Part model, mm, in its own coordinate system. Face numbers are marked on the shaded views. A direction names the side the tool comes from. Give positions to 0.01 mm unless a question says otherwise; leave off trailing zeros. Order: outer loops, then holes, each group sorted by start corner. A loop starts at its lowest first (then second) coordinate and runs counter-clockwise, first axis right, second up. Notation, with made-up numbers: (20.25, -6) - (27.25, -6) arc R20 cw to (27.25, 15) - close; hole circle Ø2 at (-33, 80). An arc over 180 degrees is marked (long way). Use a Markdown table: item, result. Add a question column.
from build123d import *

# Parameters (mm, degrees)
SKETCH1_R           = 127
BOSS_EXTRUDE1_DEPTH = 63.5
BOSS_EXTRUDE2_DEPTH = 381
CUT_EXTRUDE1_DEPTH  = 203.2
CUT_EXTRUDE2_DEPTH  = 203.2
FILLET1_R           = 25.4
FILLET2_R           = 25.4
FILLET3_R           = 25.4
SKETCH5_R           = 127
BOSS_EXTRUDE3_DEPTH = 304.8
SKETCH6_R           = 63.5
BOSS_EXTRUDE4_DEPTH = 127


with BuildPart() as part:
    # Sketch1 → Boss-Extrude1 (new body, symmetric)
    with BuildSketch(Plane(origin=(0, 0, 0), x_dir=(0, 0, -1), z_dir=(1, 0, 0))):
        Circle(SKETCH1_R)
    extrude(amount=BOSS_EXTRUDE1_DEPTH, both=True)

    # Sketch2 → Boss-Extrude2 (add, symmetric)
    with BuildSketch(Plane.XY):
        Polygon((88.9, -120.65), (88.9, 120.65), (317.5, 158.75), (311.236398584, 196.331608498), (50.8, 152.925542067), (50.8, -152.925542067), (311.236398584, -196.331608498), (317.5, -158.75), align=None)
    extrude(amount=BOSS_EXTRUDE2_DEPTH, both=True)

    # Sketch3 → Cut-Extrude1 (cut)
    with BuildSketch(Plane(origin=(334.662162162, 55.777027027, 0), x_dir=(0, 0, -1), z_dir=(0.986393924, 0.164398987, 0))):
        Polygon((0, 104.393356939), (-127, 104.393356939), (-127, 142.493356939), (127, 142.493356939), (127, 104.393356939), align=None)
    extrude(amount=-CUT_EXTRUDE1_DEPTH, mode=Mode.SUBTRACT)

    # Sketch4 → Cut-Extrude2 (cut)
    with BuildSketch(Plane(origin=(334.662162162, -55.777027027, 0), x_dir=(0, 0, -1), z_dir=(0.986393924, -0.164398987, 0))):
        Polygon((0, -142.493356939), (-127, -142.493356939), (-127, -104.393356939), (127, -104.393356939), (127, -142.493356939), align=None)
    extrude(amount=-CUT_EXTRUDE2_DEPTH, mode=Mode.SUBTRACT)

    # Fillet1
    fillet1_edges = [part.edges().sort_by_distance(p)[0] for p in [
        (88.9, -120.65, 0),
        (88.9, 120.65, 0),
    ]]
    fillet(fillet1_edges, radius=FILLET1_R)

    # Fillet2
    fillet2_edges = [part.edges().sort_by_distance(p)[0] for p in [
        (50.8, 152.925542067, 0),
        (50.8, -152.925542067, 0),
    ]]
    fillet(fillet2_edges, radius=FILLET2_R)

    # Fillet3
    fillet3_edges = [part.edges().sort_by_distance(p)[0] for p in [
        (314.368199292, -177.540804249, 381),
        (113.932953969, 144.134930029, 127),
        (113.932953969, 144.134930029, -127),
        (314.368199292, 177.540804249, -127),
        (314.368199292, 177.540804249, 127),
        (113.932953969, -144.134930029, 127),
        (113.932953969, -144.134930029, -127),
        (314.368199292, -177.540804249, -127),
        (314.368199292, -177.540804249, 127),
        (314.368199292, 177.540804249, -381),
        (314.368199292, -177.540804249, -381),
        (314.368199292, 177.540804249, 381),
    ]]
    fillet(fillet3_edges, radius=FILLET3_R)

    # Sketch5 → Boss-Extrude3 (add)
    with BuildSketch(Plane.ZY.offset(63.5)):
        Circle(SKETCH5_R)
    extrude(amount=BOSS_EXTRUDE3_DEPTH)

    # Sketch6 → Boss-Extrude4 (add)
    with BuildSketch(Plane.ZY.offset(368.3)):
        Circle(SKETCH6_R)
    extrude(amount=BOSS_EXTRUDE4_DEPTH)


solid = part.part
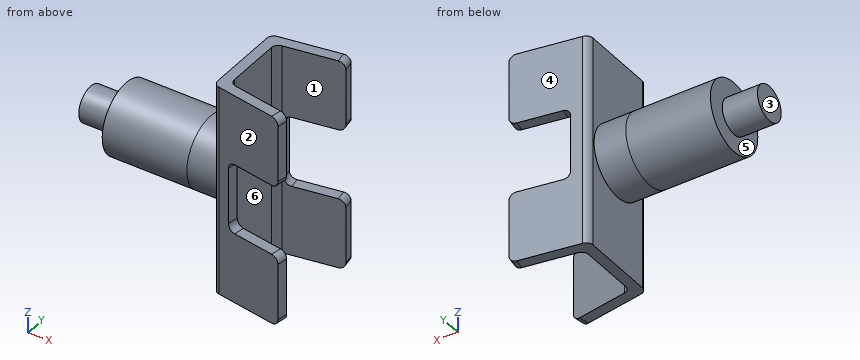
1. Mould opens along Y. For the marked faces 1, 2 and 3 say: released by +Y, released by -Y, zero draft, split by the parting line, or undercut.
2. Pin check, flat tips, straight feed: P1, Ø5, axis at x = -244.5, y = 65.5, coming from the -Z side; P2, Ø3, axis at y = -11, z = 181, coming from the +X side; P3, Ø6, axis at x = 181.5, z = 247.5, coming from the -Y side. Stop position of each tip, or through.
3. Cut at D-D (x = -27.5). Write the cut outline in (y, z).
4. Tool access for the marked faces 4, 5 and 6: list every direction of +Z, -Z, +X, -X, +Y, -Y with a clear straight run to the whole face (end or side of a thin tool).
5. Cut at B-B (y = 0). Write the cut outline in (x, z).
6. Drill centre lines: probe 1 along X at (y, z) = (-31.5, 104.5); probe 2 along Y at (x, z) = (197.5, -225); probe 3 along X at (y, z) = (42.5, -283.5). Where is each one in solid material? Low to high. Write a range as [from, to].
7. Cut at A-A (x = 99). Write the cut outline in (y, z).
8. Cut at C-C (z = -295.5). Write the cut outline in (x, y), plus the area to 3 significant figures.
Responses:
| question | item | result |
|---|---|---|
| 1 | face 1 | undercut |
| 1 | face 2 | released by -Y |
| 1 | face 3 | zero draft |
| 2 | P1 | stops at z = -110.27 |
| 2 | P2 | stops at x = 88.9 |
| 2 | P3 | stops at y = -175.21 |
| 3 | outline | circle Ø254 at (0, 0) |
| 4 | face 4 | +Z, -Z, -X, +Y |
| 4 | face 5 | -X |
| 4 | face 6 | +Z, -Z, +X |
| 5 | outline | (-495.3, -63.5) - (-368.3, -63.5) - (-368.3, -127) - (50.8, -127) - (50.8, -381) - (88.9, -381) - (88.9, 381) - (50.8, 381) - (50.8, 127) - (-368.3, 127) - (-368.3, 63.5) - (-495.3, 63.5) - close |
| 6 | probe 1 | x = [-368.3, 88.9] |
| 6 | probe 2 | y = [-177.38, -138.75], [138.75, 177.38] |
| 6 | probe 3 | x = [50.8, 88.9] |
| 7 | outline | (-160.96, -381) - (-119.41, -381) - (-119.41, 381) - (-160.96, 381) - close; (119.41, -381) - (160.96, -381) - (160.96, 381) - (119.41, 381) - close |
| 8 | outline | (50.8, -131.41) arc R25.4 ccw to (72.02, -156.46) - (311.24, -196.33) - (317.5, -158.75) - (110.12, -124.19) arc R25.4 cw to (88.9, -99.13) - (88.9, 99.13) arc R25.4 cw to (110.12, 124.19) - (317.5, 158.75) - (311.24, 196.33) - (72.02, 156.46) arc R25.4 ccw to (50.8, 131.41) - close |
| 8 | area | 29,300 mm² |
